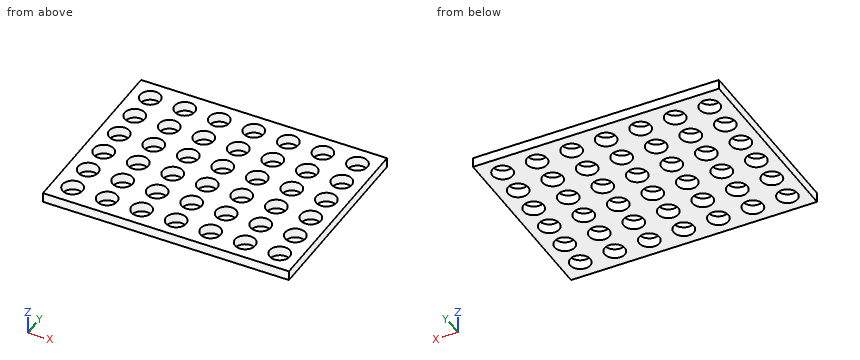
```python
from build123d import *

# Parameters (mm, degrees)
SKETCH_W  = 63.340006
SKETCH_H  = 48.1
SKETCH_R  = 2.6
PAD_DEPTH = 2.5


with BuildPart() as part:
    # Sketch → Pad (new body)
    with BuildSketch(Plane.XY):
        with Locations((31.670003, 24.05)):
            Rectangle(SKETCH_W, SKETCH_H)
        with Locations((5, 43.1)):
            Circle(SKETCH_R, mode=Mode.SUBTRACT)
        with Locations((13.890001, 43.1)):
            Circle(SKETCH_R, mode=Mode.SUBTRACT)
        with Locations((22.780002, 43.1)):
            Circle(SKETCH_R, mode=Mode.SUBTRACT)
        with Locations((31.670003, 43.1)):
            Circle(SKETCH_R, mode=Mode.SUBTRACT)
        with Locations((40.560004, 43.1)):
            Circle(SKETCH_R, mode=Mode.SUBTRACT)
        with Locations((49.450005, 43.1)):
            Circle(SKETCH_R, mode=Mode.SUBTRACT)
        with Locations((58.340006, 43.1)):
            Circle(SKETCH_R, mode=Mode.SUBTRACT)
        with Locations((5, 35.48)):
            Circle(SKETCH_R, mode=Mode.SUBTRACT)
        with Locations((13.890001, 35.48)):
            Circle(SKETCH_R, mode=Mode.SUBTRACT)
        with Locations((22.780002, 35.48)):
            Circle(SKETCH_R, mode=Mode.SUBTRACT)
        with Locations((31.670003, 35.48)):
            Circle(SKETCH_R, mode=Mode.SUBTRACT)
        with Locations((40.560004, 35.48)):
            Circle(SKETCH_R, mode=Mode.SUBTRACT)
        with Locations((49.450005, 35.48)):
            Circle(SKETCH_R, mode=Mode.SUBTRACT)
        with Locations((58.340006, 35.48)):
            Circle(SKETCH_R, mode=Mode.SUBTRACT)
        with Locations((5, 27.86)):
            Circle(SKETCH_R, mode=Mode.SUBTRACT)
        with Locations((13.890001, 27.86)):
            Circle(SKETCH_R, mode=Mode.SUBTRACT)
        with Locations((22.780002, 27.86)):
            Circle(SKETCH_R, mode=Mode.SUBTRACT)
        with Locations((31.670003, 27.86)):
            Circle(SKETCH_R, mode=Mode.SUBTRACT)
        with Locations((40.560004, 27.86)):
            Circle(SKETCH_R, mode=Mode.SUBTRACT)
        with Locations((49.450005, 27.86)):
            Circle(SKETCH_R, mode=Mode.SUBTRACT)
        with Locations((58.340006, 27.86)):
            Circle(SKETCH_R, mode=Mode.SUBTRACT)
        with Locations((5, 20.24)):
            Circle(SKETCH_R, mode=Mode.SUBTRACT)
        with Locations((13.890001, 20.24)):
            Circle(SKETCH_R, mode=Mode.SUBTRACT)
        with Locations((22.780002, 20.24)):
            Circle(SKETCH_R, mode=Mode.SUBTRACT)
        with Locations((31.670003, 20.24)):
            Circle(SKETCH_R, mode=Mode.SUBTRACT)
        with Locations((40.560004, 20.24)):
            Circle(SKETCH_R, mode=Mode.SUBTRACT)
        with Locations((49.450005, 20.24)):
            Circle(SKETCH_R, mode=Mode.SUBTRACT)
        with Locations((58.340006, 20.24)):
            Circle(SKETCH_R, mode=Mode.SUBTRACT)
        with Locations((5, 12.62)):
            Circle(SKETCH_R, mode=Mode.SUBTRACT)
        with Locations((13.890001, 12.62)):
            Circle(SKETCH_R, mode=Mode.SUBTRACT)
        with Locations((22.780002, 12.62)):
            Circle(SKETCH_R, mode=Mode.SUBTRACT)
        with Locations((31.670003, 12.62)):
            Circle(SKETCH_R, mode=Mode.SUBTRACT)
        with Locations((40.560004, 12.62)):
            Circle(SKETCH_R, mode=Mode.SUBTRACT)
        with Locations((49.450005, 12.62)):
            Circle(SKETCH_R, mode=Mode.SUBTRACT)
        with Locations((58.340006, 12.62)):
            Circle(SKETCH_R, mode=Mode.SUBTRACT)
        with Locations((5, 5)):
            Circle(SKETCH_R, mode=Mode.SUBTRACT)
        with Locations((13.890001, 5)):
            Circle(SKETCH_R, mode=Mode.SUBTRACT)
        with Locations((22.780002, 5)):
            Circle(SKETCH_R, mode=Mode.SUBTRACT)
        with Locations((31.670003, 5)):
            Circle(SKETCH_R, mode=Mode.SUBTRACT)
        with Locations((40.560004, 5)):
            Circle(SKETCH_R, mode=Mode.SUBTRACT)
        with Locations((49.450005, 5)):
            Circle(SKETCH_R, mode=Mode.SUBTRACT)
        with Locations((58.340006, 5)):
            Circle(SKETCH_R, mode=Mode.SUBTRACT)
    extrude(amount=PAD_DEPTH)


solid = part.part
```
Geometry: final body of the model. Coordinates: model frame, mm. Coordinates: 2 decimals unless noted, no trailing zeros. Order: outer loops, then holes, each group sorted by start corner. A loop starts at its lowest first (then second) coordinate and runs counter-clockwise, first axis right, second up. Notation, with made-up numbers: (15.25, -35.75) -> (58.25, -35.75) arc R18 ccw to (58.25, -19.75) -> close; hole circle Ø3 at (-14.75, 53.5). An arc over 180 degrees is marked (long way). Use CSV: the item, a comma, the result in double quotes.
1) Section A-A on y = 5. State how many separate pieces and enclosed holes the cut face has, then the cut area to 4 significant figures.
Findings:
separate pieces,"8"
enclosed holes,"0"
area,"67.35 mm^2"
2) Section B-B on x = 13.89. Output: boundary loops of the cut face in (y, z), then the cut area to 4 significant figures.
Findings:
outline,"(0, 0) -> (2.4, 0) -> (2.4, 2.5) -> (0, 2.5) -> close; (7.6, 0) -> (10.02, 0) -> (10.02, 2.5) -> (7.6, 2.5) -> close; (15.22, 0) -> (17.64, 0) -> (17.64, 2.5) -> (15.22, 2.5) -> close; (22.84, 0) -> (25.26, 0) -> (25.26, 2.5) -> (22.84, 2.5) -> close; (30.46, 0) -> (32.88, 0) -> (32.88, 2.5) -> (30.46, 2.5) -> close; (38.08, 0) -> (40.5, 0) -> (40.5, 2.5) -> (38.08, 2.5) -> close; (45.7, 0) -> (48.1, 0) -> (48.1, 2.5) -> (45.7, 2.5) -> close"
area,"42.25 mm^2"
3) Pin query (flat end, axial travel): pin 1 Ø4.5 at (x, y) = (58.34, 35.48) entering from -Z. Return the tip coordinate at first contact, or that it passes through.
Findings:
pin 1,"passes through"
4) Section D-D on x = 21. Output: boundary loops of the cut face in (y, z), then the cut area to 3 significant figures.
Findings:
outline,"(0, 0) -> (3.1, 0) -> (3.1, 2.5) -> (0, 2.5) -> close; (6.9, 0) -> (10.72, 0) -> (10.72, 2.5) -> (6.9, 2.5) -> close; (14.52, 0) -> (18.34, 0) -> (18.34, 2.5) -> (14.52, 2.5) -> close; (22.14, 0) -> (25.96, 0) -> (25.96, 2.5) -> (22.14, 2.5) -> close; (29.76, 0) -> (33.58, 0) -> (33.58, 2.5) -> (29.76, 2.5) -> close; (37.38, 0) -> (41.2, 0) -> (41.2, 2.5) -> (37.38, 2.5) -> close; (45, 0) -> (48.1, 0) -> (48.1, 2.5) -> (45, 2.5) -> close"
area,"63.4 mm^2"
